from build123d import *

# Parameters (mm, degrees)
SKETCH1_R           = 1.2
SKETCH1_R_2         = 4.4
BOSS_EXTRUDE1_DEPTH = 4
SKETCH3_W           = 34
SKETCH3_H           = 46
SKETCH3_R           = 5
SKETCH3_R_2         = 1.7
BOSS_EXTRUDE3_DEPTH = 4


with BuildPart() as part:
    # Sketch1 → Boss-Extrude1 (new body)
    with BuildSketch(Plane.XY):
        with BuildLine():
            Line((-10.25, -28.75), (10.25, -28.75))
            Line((10.25, -28.75), (10.25, 0))
            ThreePointArc((10.25, 0), (0, 10.25), (-10.25, 0))
            Line((-10.25, 0), (-10.25, -28.75))
        make_face()
        with Locations((0, 8)):
            Circle(SKETCH1_R, mode=Mode.SUBTRACT)
        with Locations((-8, 0)):
            Circle(SKETCH1_R, mode=Mode.SUBTRACT)
        with Locations((0, -8)):
            Circle(SKETCH1_R, mode=Mode.SUBTRACT)
        with Locations((8, 0)):
            Circle(SKETCH1_R, mode=Mode.SUBTRACT)
        Circle(SKETCH1_R_2, mode=Mode.SUBTRACT)
    boss_extrude1 = extrude(amount=BOSS_EXTRUDE1_DEPTH)

    # Sketch3 → Boss-Extrude3 (add)
    with BuildSketch(Plane(origin=(0, -28.75, 0), x_dir=(-1, 0, 0), z_dir=(0, -1, 0))):
        with Locations((0, -23)):
            Rectangle(SKETCH3_W, SKETCH3_H)
        with Locations(Location((0, -23, 0), (0, 0, 180))):
            Circle(SKETCH3_R, mode=Mode.SUBTRACT)
        with Locations(Location((-8.25, -14, 0), (0, 0, 180))):
            Circle(SKETCH3_R_2, mode=Mode.SUBTRACT)
        with Locations(Location((8.25, -14, 0), (0, 0, 180))):
            Circle(SKETCH3_R_2, mode=Mode.SUBTRACT)
        with Locations(Location((8.25, -32, 0), (0, 0, 180))):
            Circle(SKETCH3_R_2, mode=Mode.SUBTRACT)
        with Locations(Location((-8.25, -32, 0), (0, 0, 180))):
            Circle(SKETCH3_R_2, mode=Mode.SUBTRACT)
    extrude(amount=-BOSS_EXTRUDE3_DEPTH)

    # Mirror1: Boss-Extrude1 across plane
    add(boss_extrude1.mirror(Plane.XY.offset(23)))


solid = part.part
For this review, take the finished solid that the model builds, in its own axes (mm). A direction names the side the tool comes from. Round coordinates to 2 decimals unless told otherwise and drop trailing zeros. Order: outer loops, then holes, each group sorted by start corner. A loop starts at its lowest first (then second) coordinate and runs counter-clockwise, first axis right, second up. Notation, with made-up numbers: (-8.75, 73.25) -> (20.25, 73.25) arc R27 cw to (20.25, 94.25) -> close; hole circle Ø9 at (49.5, 0.25). An arc over 180 degrees is marked (long way). Write item = value, one per line. Start each with the question number.
1) Take a section at C-C on x = -8.25. State the section outline as (y, z) points, plus the area to 3 significant figures.
2) Insertion check: pin 1 (3 mm diameter, centred on y = -15, z = 1, fed in from +X); pin 2 (6 mm diameter, centred on x = -13, z = 11.5, fed in from +Y); pin 3 (4 mm diameter, centred on x = -1, y = -0.5, fed in from -Z); pin 4 (4.5 mm diameter, centred on y = -13, z = 45, fed in from -X). Each pin has a flat end and moves straight along its axis. Give the tip position at first contact, or say it passes through.
3) Take a section at D-D on y = -2. State the section outline as (x, z) points.
4) Tool access review of faces 1 (the face through (-10.25, -12, 44)), 2 (the face through (0, -14, 0)), 3 (the face through (0, -11, 42)): name each direction out of +Z, -Z, +X, -X, +Y, -Y from which nothing blocks a thin tool from reaching the whole face with its end or side.
5) Take a section at A-A on y = -8. State the section outline as (x, z) points.
6) Take a section at B-B on z = 23. State the section outline as (x, y) points.
7) To check wall thickness, follow line 1 (Z direction, x = -8.25, y = -25.85); line 2 (Y direction, x = 0, z = 3); line 3 (Z direction, x = 5, y = -7). State the ranges of each line that lie inside material, in increasing order. Write a range as from..to.
8) The part is to be moulded in two halves that separate along Z. For faces 4 (the face through (0, -14, 46)), 5 (the face through (-17, -27, 23)), 6 (the face through (0.2, -24.75, 17.6)), 7 (the face through (-1.08, -26.78, 18.12)), say which applies: +Z half, -Z half, draft (parallel to the pull), parting line (faces both ways), or undercut.
Verdict:
q1.outline = (-28.75, 0) -> (-1.17, 0) -> (-1.17, 4) -> (-24.75, 4) -> (-24.75, 12.3) -> (-28.75, 12.3) -> close; (-28.75, 15.7) -> (-24.75, 15.7) -> (-24.75, 30.3) -> (-28.75, 30.3) -> close; (-28.75, 33.7) -> (-24.75, 33.7) -> (-24.75, 42) -> (-1.17, 42) -> (-1.17, 46) -> (-28.75, 46) -> close; (1.17, 0) -> (6.08, 0) -> (6.08, 4) -> (1.17, 4) -> close; (1.17, 42) -> (6.08, 42) -> (6.08, 46) -> (1.17, 46) -> close
q1.area = 385 mm2
q2.pin_1 = 10.25
q2.pin_2 = -24.75
q2.pin_3 = through
q2.pin_4 = -10.25
q3.outline = (-10.25, 0) -> (-3.92, 0) -> (-3.92, 4) -> (-10.25, 4) -> close; (-10.25, 42) -> (-3.92, 42) -> (-3.92, 46) -> (-10.25, 46) -> close; (3.92, 0) -> (10.25, 0) -> (10.25, 4) -> (3.92, 4) -> close; (3.92, 42) -> (10.25, 42) -> (10.25, 46) -> (3.92, 46) -> close
q4.face_1 = +Z, -Z, -X, +Y
q4.face_2 = -Z, +X, -X, +Y, -Y
q4.face_3 = +X, -X, +Y
q5.outline = (-10.25, 0) -> (-1.2, 0) -> (-1.2, 4) -> (-10.25, 4) -> close; (-10.25, 42) -> (-1.2, 42) -> (-1.2, 46) -> (-10.25, 46) -> close; (1.2, 0) -> (10.25, 0) -> (10.25, 4) -> (1.2, 4) -> close; (1.2, 42) -> (10.25, 42) -> (10.25, 46) -> (1.2, 46) -> close
q6.outline = (-17, -28.75) -> (-5, -28.75) -> (-5, -24.75) -> (-17, -24.75) -> close; (5, -28.75) -> (17, -28.75) -> (17, -24.75) -> (5, -24.75) -> close
q7.line_1 = 0..12.3, 15.7..30.3, 33.7..46
q7.line_2 = -28.75..-9.2, -6.8..-4.4, 4.4..6.8, 9.2..10.25
q7.line_3 = 0..4, 42..46
q8.face_4 = +Z half
q8.face_5 = draft
q8.face_6 = undercut
q8.face_7 = undercut
